from build123d import *

# Parameters (mm, degrees)
SKETCH_1_R      = 1.5
SKETCH_1_W      = 5
SKETCH_1_H      = 20
SKETCH_1_W_2    = 20
SKETCH_1_H_2    = 5
EXTRUDE_1_DEPTH = 5


with BuildPart() as part:
    # 草图1 → 凸台-拉伸1 (new body)
    with BuildSketch(Plane(origin=(0, 0, 0), x_dir=(0, 0, -1), z_dir=(1, 0, 0))):
        with BuildLine():
            Line((-75.770893239, -36.323671614), (-75.770893239, -33.323671614))
            ThreePointArc((-75.770893239, -33.323671614), (-75.185106801, -31.909458051), (-73.770893239, -31.323671614))
            Line((-73.770893239, -31.323671614), (162.229106761, -31.323671614))
            ThreePointArc((162.229106761, -31.323671614), (163.643320323, -31.909458051), (164.229106761, -33.323671614))
            Line((164.229106761, -33.323671614), (164.229106761, -36.323671614))
            ThreePointArc((164.229106761, -36.323671614), (165.693572855, -39.85920552), (169.229106761, -41.323671614))
            Line((169.229106761, -41.323671614), (209.229106761, -41.323671614))
            ThreePointArc((209.229106761, -41.323671614), (212.764640667, -39.85920552), (214.229106761, -36.323671614))
            Line((214.229106761, -36.323671614), (214.229106761, -4.023671614))
            Line((214.229106761, -4.023671614), (219.229106761, -4.023671614))
            Line((219.229106761, -4.023671614), (219.229106761, 15.976328386))
            Line((219.229106761, 15.976328386), (214.229106761, 15.976328386))
            Line((214.229106761, 15.976328386), (214.229106761, 24.476328386))
            Line((214.229106761, 24.476328386), (211.229106761, 24.476328386))
            Line((211.229106761, 24.476328386), (211.229106761, 23.226328386))
            Line((211.229106761, 23.226328386), (208.229106761, 23.226328386))
            Line((208.229106761, 23.226328386), (208.229106761, 24.476328386))
            Line((208.229106761, 24.476328386), (206.229106761, 24.476328386))
            Line((206.229106761, 24.476328386), (206.229106761, 27.476328386))
            Line((206.229106761, 27.476328386), (208.229106761, 27.476328386))
            Line((208.229106761, 27.476328386), (208.229106761, 28.726328386))
            Line((208.229106761, 28.726328386), (211.229106761, 28.726328386))
            Line((211.229106761, 28.726328386), (211.229106761, 27.476328386))
            Line((211.229106761, 27.476328386), (214.229106761, 27.476328386))
            Line((214.229106761, 27.476328386), (214.229106761, 35.976328386))
            Line((214.229106761, 35.976328386), (219.229106761, 35.976328386))
            Line((219.229106761, 35.976328386), (219.229106761, 55.976328386))
            Line((219.229106761, 55.976328386), (214.229106761, 55.976328386))
            Line((214.229106761, 55.976328386), (214.229106761, 64.476328386))
            Line((214.229106761, 64.476328386), (211.229106761, 64.476328386))
            Line((211.229106761, 64.476328386), (211.229106761, 63.226328386))
            Line((211.229106761, 63.226328386), (208.229106761, 63.226328386))
            Line((208.229106761, 63.226328386), (208.229106761, 64.476328386))
            Line((208.229106761, 64.476328386), (206.229106761, 64.476328386))
            Line((206.229106761, 64.476328386), (206.229106761, 67.476328386))
            Line((206.229106761, 67.476328386), (208.229106761, 67.476328386))
            Line((208.229106761, 67.476328386), (208.229106761, 68.726328386))
            Line((208.229106761, 68.726328386), (211.229106761, 68.726328386))
            Line((211.229106761, 68.726328386), (211.229106761, 67.476328386))
            Line((211.229106761, 67.476328386), (214.229106761, 67.476328386))
            Line((214.229106761, 67.476328386), (214.229106761, 75.976328386))
            Line((214.229106761, 75.976328386), (-125.770893239, 75.976328386))
            Line((-125.770893239, 75.976328386), (-125.770893239, 67.476328386))
            Line((-125.770893239, 67.476328386), (-122.770893239, 67.476328386))
            Line((-122.770893239, 67.476328386), (-122.770893239, 68.726328386))
            Line((-122.770893239, 68.726328386), (-119.770893239, 68.726328386))
            Line((-119.770893239, 68.726328386), (-119.770893239, 67.476328386))
            Line((-119.770893239, 67.476328386), (-117.770893239, 67.476328386))
            Line((-117.770893239, 67.476328386), (-117.770893239, 64.476328386))
            Line((-117.770893239, 64.476328386), (-119.770893239, 64.476328386))
            Line((-119.770893239, 64.476328386), (-119.770893239, 63.226328386))
            Line((-119.770893239, 63.226328386), (-122.770893239, 63.226328386))
            Line((-122.770893239, 63.226328386), (-122.770893239, 64.476328386))
            Line((-122.770893239, 64.476328386), (-125.770893239, 64.476328386))
            Line((-125.770893239, 64.476328386), (-125.770893239, 55.976328386))
            Line((-125.770893239, 55.976328386), (-130.770893239, 55.976328386))
            Line((-130.770893239, 55.976328386), (-130.770893239, 35.976328386))
            Line((-130.770893239, 35.976328386), (-125.770893239, 35.976328386))
            Line((-125.770893239, 35.976328386), (-125.770893239, 27.476328386))
            Line((-125.770893239, 27.476328386), (-122.770893239, 27.476328386))
            Line((-122.770893239, 27.476328386), (-122.770893239, 28.726328386))
            Line((-122.770893239, 28.726328386), (-119.770893239, 28.726328386))
            Line((-119.770893239, 28.726328386), (-119.770893239, 27.476328386))
            Line((-119.770893239, 27.476328386), (-117.770893239, 27.476328386))
            Line((-117.770893239, 27.476328386), (-117.770893239, 24.476328386))
            Line((-117.770893239, 24.476328386), (-119.770893239, 24.476328386))
            Line((-119.770893239, 24.476328386), (-119.770893239, 23.226328386))
            Line((-119.770893239, 23.226328386), (-122.770893239, 23.226328386))
            Line((-122.770893239, 23.226328386), (-122.770893239, 24.476328386))
            Line((-122.770893239, 24.476328386), (-125.770893239, 24.476328386))
            Line((-125.770893239, 24.476328386), (-125.770893239, 15.976328386))
            Line((-125.770893239, 15.976328386), (-130.770893239, 15.976328386))
            Line((-130.770893239, 15.976328386), (-130.770893239, -4.023671614))
            Line((-130.770893239, -4.023671614), (-125.770893239, -4.023671614))
            Line((-125.770893239, -4.023671614), (-125.770893239, -36.323671614))
            ThreePointArc((-125.770893239, -36.323671614), (-124.306427145, -39.85920552), (-120.770893239, -41.323671614))
            Line((-120.770893239, -41.323671614), (-80.770893239, -41.323671614))
            ThreePointArc((-80.770893239, -41.323671614), (-77.235359333, -39.85920552), (-75.770893239, -36.323671614))
        make_face()
        with Locations((54.729106761, 25.976328386)):
            Circle(SKETCH_1_R, mode=Mode.SUBTRACT)
        with Locations((-65.270893239, 25.976328386)):
            Circle(SKETCH_1_R, mode=Mode.SUBTRACT)
        with Locations((54.729106761, 45.976328386)):
            Rectangle(SKETCH_1_W, SKETCH_1_H, mode=Mode.SUBTRACT)
        with Locations((54.729106761, 5.976328386)):
            Rectangle(SKETCH_1_W, SKETCH_1_H, mode=Mode.SUBTRACT)
        with Locations((-65.270893239, 45.976328386)):
            Rectangle(SKETCH_1_W, SKETCH_1_H, mode=Mode.SUBTRACT)
        with Locations((-65.270893239, 5.976328386)):
            Rectangle(SKETCH_1_W, SKETCH_1_H, mode=Mode.SUBTRACT)
        with Locations((-25.770893239, -23.823671614)):
            Rectangle(SKETCH_1_W_2, SKETCH_1_H_2, mode=Mode.SUBTRACT)
        with Locations((-95.770893239, -23.823671614)):
            Rectangle(SKETCH_1_W_2, SKETCH_1_H_2, mode=Mode.SUBTRACT)
        with Locations((194.229106761, -23.823671614)):
            Rectangle(SKETCH_1_W_2, SKETCH_1_H_2, mode=Mode.SUBTRACT)
        with Locations((144.229106761, -23.823671614)):
            Rectangle(SKETCH_1_W_2, SKETCH_1_H_2, mode=Mode.SUBTRACT)
        with BuildLine():
            Line((191.229106761, 18.676328386), (147.229106761, 18.676328386))
            ThreePointArc((147.229106761, 18.676328386), (141.572252511, 16.333182636), (139.229106761, 10.676328386))
            Line((139.229106761, 10.676328386), (139.229106761, -8.323671614))
            ThreePointArc((139.229106761, -8.323671614), (141.572252511, -13.980525863), (147.229106761, -16.323671614))
            Line((147.229106761, -16.323671614), (191.229106761, -16.323671614))
            ThreePointArc((191.229106761, -16.323671614), (196.88596101, -13.980525863), (199.229106761, -8.323671614))
            Line((199.229106761, -8.323671614), (199.229106761, 10.676328386))
            ThreePointArc((199.229106761, 10.676328386), (196.88596101, 16.333182636), (191.229106761, 18.676328386))
        make_face(mode=Mode.SUBTRACT)
        with BuildLine():
            Line((82.229106761, 55.976328386), (77.229106761, 55.976328386))
            ThreePointArc((77.229106761, 55.976328386), (73.693572855, 54.511862292), (72.229106761, 50.976328386))
            Line((72.229106761, 50.976328386), (72.229106761, 0.976328386))
            ThreePointArc((72.229106761, 0.976328386), (73.693572855, -2.55920552), (77.229106761, -4.023671614))
            Line((77.229106761, -4.023671614), (82.229106761, -4.023671614))
            ThreePointArc((82.229106761, -4.023671614), (85.764640667, -2.55920552), (87.229106761, 0.976328386))
            Line((87.229106761, 0.976328386), (87.229106761, 50.976328386))
            ThreePointArc((87.229106761, 50.976328386), (85.764640667, 54.511862292), (82.229106761, 55.976328386))
        make_face(mode=Mode.SUBTRACT)
        with BuildLine():
            Line((-32.770893239, 40.976328386), (-3.770893239, 40.976328386))
            ThreePointArc((-3.770893239, 40.976328386), (-1.649572896, 40.09764873), (-0.770893239, 37.976328386))
            Line((-0.770893239, 37.976328386), (-0.770893239, 33.976328386))
            ThreePointArc((-0.770893239, 33.976328386), (-1.649572896, 31.855008043), (-3.770893239, 30.976328386))
            Line((-3.770893239, 30.976328386), (-32.770893239, 30.976328386))
            ThreePointArc((-32.770893239, 30.976328386), (-34.892213583, 31.855008043), (-35.770893239, 33.976328386))
            Line((-35.770893239, 33.976328386), (-35.770893239, 37.976328386))
            ThreePointArc((-35.770893239, 37.976328386), (-34.892213583, 40.09764873), (-32.770893239, 40.976328386))
        make_face(mode=Mode.SUBTRACT)
    extrude(amount=EXTRUDE_1_DEPTH)


solid = part.part
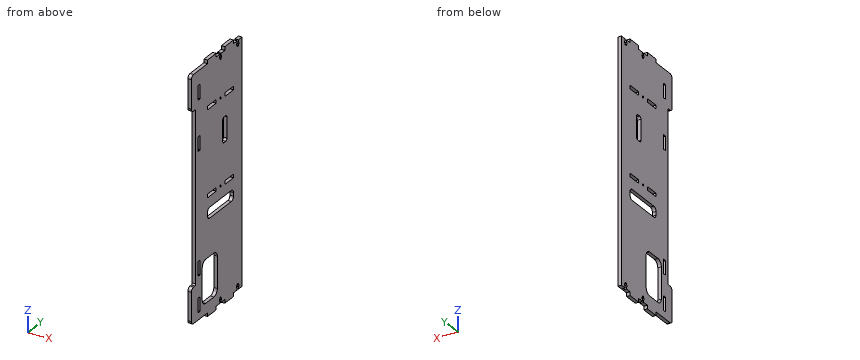
Check sheet for the modelled part. Datum: model origin and axes. Units: mm. Give positions to 0.01 mm unless a question says otherwise; leave off trailing zeros. Order: outer loops, then holes, each group sorted by start corner. A loop starts at its lowest first (then second) coordinate and runs counter-clockwise, first axis right, second up. Notation, with made-up numbers: M -12.5,80.5 L 40.5,80.5 A36 cw 40.5,119.5 Z; hole C 13.5,43.5 d7. An arc over 180 degrees is marked long. Answer as CSV lines item,"result". Start each with the question number.
Item 1: Gauge pin test, flat ends, axial feed: P1, Ø0.6, axis at x = 2, y = 63.5, coming from the +Z side; P2, Ø8, axis at y = 41.5, z = 15, coming from the -X side; P3, Ø1.5, axis at x = 2, z = -79, coming from the -Y side; P4, Ø0.6, axis at x = 2.5, y = 68.5, coming from the -Z side. Record the tip position at first contact, or that the pin passes through.
Item 2: Cross-section at B-B on x = 1.9. State how many separate pieces and enclosed holes the cut face has, plus the area to 3 significant figures.
Item 3: Thickness scan on line 1 (Z direction, x = 2.05, y = 43); line 2 (Z direction, x = 0.6, y = 37.5); line 3 (Z direction, x = 2.1, y = 34). Record the ranges inside material, lowest first. Write a range as [from, to].
Item 4: Cross-section at A-A on z = -97. Enter the section's corners in (x, y), plus the area to 4 significant figures.
Established:
1,P1,"stops at z = 125.77"
1,P2,"stops at x = 0"
1,P3,"stops at y = -31.32"
1,P4,"stops at z = -214.23"
2,separate pieces,"1"
2,enclosed holes,"13"
2,area,"33,700 mm^2"
3,line 1,"z = [-219.23, -87.23], [-72.23, -57.23], [-52.23, 62.77], [67.77, 130.77]"
3,line 2,"z = [-219.23, -87.23], [-72.23, -57.23], [-52.23, 0.77], [35.77, 62.77], [67.77, 130.77]"
3,line 3,"z = [-214.23, -87.23], [-72.23, 0.77], [35.77, 125.77]"
4,outline,"M 0,-31.32 L 5,-31.32 L 5,75.98 L 0,75.98 Z"
4,area,"536.5 mm^2"
